Check sheet for the modelled part. Datum: model origin and axes. Units: mm. A direction names the side the tool comes from. Coordinates: 2 decimals unless noted, no trailing zeros. Order: outer loops, then holes, each group sorted by start corner. A loop starts at its lowest first (then second) coordinate and runs counter-clockwise, first axis right, second up.
from build123d import *

# Parameters (mm, degrees)
SKETCH1_R      = 4.7625
EXTRUDE1_DEPTH = 38.1
EXTRUDE2_DEPTH = 6.35
SKETCH4_W      = 11.994523233
SKETCH4_H      = 10.10814551
EXTRUDE4_DEPTH = 0.508
EXTRUDE5_DEPTH = 1.27


with BuildPart() as part:
    # Sketch1 → Extrude1 (new body)
    with BuildSketch(Plane.XY):
        Circle(SKETCH1_R)
    extrude(amount=EXTRUDE1_DEPTH)

    # Sketch2 → Extrude2 (cut)
    with BuildSketch(Plane.XY.offset(38.1)):
        with BuildLine():
            Line((-0.7112, 3.302), (1.27, 3.302))
            Line((1.27, 3.302), (1.27, 10.556011527))
            Line((1.27, 10.556011527), (23.809552604, 10.556011527))
            Line((23.809552604, 10.556011527), (23.809552604, -10.556011527))
            Line((23.809552604, -10.556011527), (1.27, -10.556011527))
            Line((1.27, -10.556011527), (1.27, -3.302))
            Line((1.27, -3.302), (-0.7112, -3.302))
            ThreePointArc((-0.7112, -3.302), (-1.555344075, -2.952344075), (-1.905, -2.1082))
            Line((-1.905, -2.1082), (-1.905, 2.1082))
            ThreePointArc((-1.905, 2.1082), (-1.555344075, 2.952344075), (-0.7112, 3.302))
        make_face()
    extrude(amount=-EXTRUDE2_DEPTH, mode=Mode.SUBTRACT)

    # Sketch4 → Extrude4 (cut)
    with BuildSketch(Plane.XY.offset(38.1)):
        with Locations((-0.260671281, -1.752072755)):
            Rectangle(SKETCH4_W, SKETCH4_H)
    extrude(amount=-EXTRUDE4_DEPTH, mode=Mode.SUBTRACT)

    # Sketch5 → Extrude5 (cut)
    with BuildSketch(Plane(origin=(1.27, 0, 0), x_dir=(0, 0, -1), z_dir=(1, 0, 0))):
        Polygon((-36.83, 5.902578594), (-36.83, -11.457674659), (-34.4424, -11.457674659), (-34.4424, 3.302), (-31.75, 3.302), (-31.75, 5.902578594), align=None)
    extrude(amount=-EXTRUDE5_DEPTH, mode=Mode.SUBTRACT)


solid = part.part
(1) Tool access check on faces 4 (the flat face through (-1, 4, 38.1)), 5 (the flat face through (0, -3.302, 34)), 6 (the flat face through (0, 4, 34)), 7 (the flat face through (1.27, -4, 33)), 8 (the flat face through (1, -4, 36.83)). Record the directions out of +Z, -Z, +X, -X, +Y, -Y that give a thin tool (end or side, any length) a straight path to the whole face; none if there is none.
Filled in:
face 4: +Z, +X, -X, +Y, -Y
face 5: +Z, +X
face 6: +X, +Y
face 7: +Z, +X, +Y, -Y
face 8: +X, +Y, -Y
(2) Thickness scan on probe 1 along Y at (x, z) = (-0.25, 36); probe 2 along Z at (x, y) = (-3.5, -0.75); probe 3 along Z at (x, y) = (3, -1.75). Record the ranges inside material, lowest first.
Filled in:
probe 1: y = -4.76 to -3.3, 3.3 to 4.76
probe 2: z = 0 to 37.59
probe 3: z = 0 to 31.75
(3) Release check for a two-part mould opening along Z. For faces 1 (the flat face through (1.27, 4, 37)), 2 (the flat face through (-2.5, -0.7, 37.592)), 3 (the flat face through (0, -4, 36)) record: +Z half, -Z half, draft (parallel to the pull), parting line (faces both ways), or undercut.
Filled in:
face 1: draft
face 2: +Z half
face 3: undercut
(4) Cross-section at D-D (y = 4). Enter the section's corners in (x, z), and give its area (3 significant figures).
Filled in:
outline: (-2.58, 0) - (2.58, 0) - (2.58, 31.75) - (0, 31.75) - (0, 36.83) - (1.27, 36.83) - (1.27, 38.1) - (-2.58, 38.1) - close
area: 182 mm2
(5) Cross-section at C-C (z = 4). Enter the section's corners in (x, y) (1 decimal), and give its area (3 significant figures).
Filled in:
outline: circle Ø9.5 at (0, 0)
area: 71.3 mm2
(6) Cross-section at B-B (x = -1.5). Enter the section's corners in (y, z).
Filled in:
outline: (-4.52, 0) - (4.52, 0) - (4.52, 38.1) - (3.3, 38.1) - (3.3, 37.59) - (3, 37.59) - (3, 31.75) - (-3, 31.75) - (-3, 37.59) - (-4.52, 37.59) - close
(7) Go/stop test with flat-tipped pins: P1, Ø3, axis at x = -3, y = -0.5, coming from the +Z side; P2, Ø1.6, axis at y = 4, z = 34, coming from the +X side; P3, Ø0.6, axis at y = 3.5, z = 37, coming from the +X side. Record where each tip stops, or that it passes through.
Filled in:
P1: stops at z = 37.59
P2: stops at x = 0
P3: stops at x = 1.27
